Geometry check sheet. Reference: drawing and pictorial views, mm from the part's lowest x, y, z. Round coordinates to 2 decimals unless told otherwise and drop trailing zeros. Write each loop counter-clockwise with the first axis right and the second up, starting at its lowest first coordinate (ties: lowest second). Pieces come first, ordered by that corner, then holes. Notation, with made-up numbers: (-8, 82.5) -> (34, 82.5) arc R20 cw to (34, 103.5) -> close; hole circle Ø11 at (27.25, 69.25). An arc over 180 degrees is marked (long way). Answer as a JSON object with one key per item and string values. Group by question number.
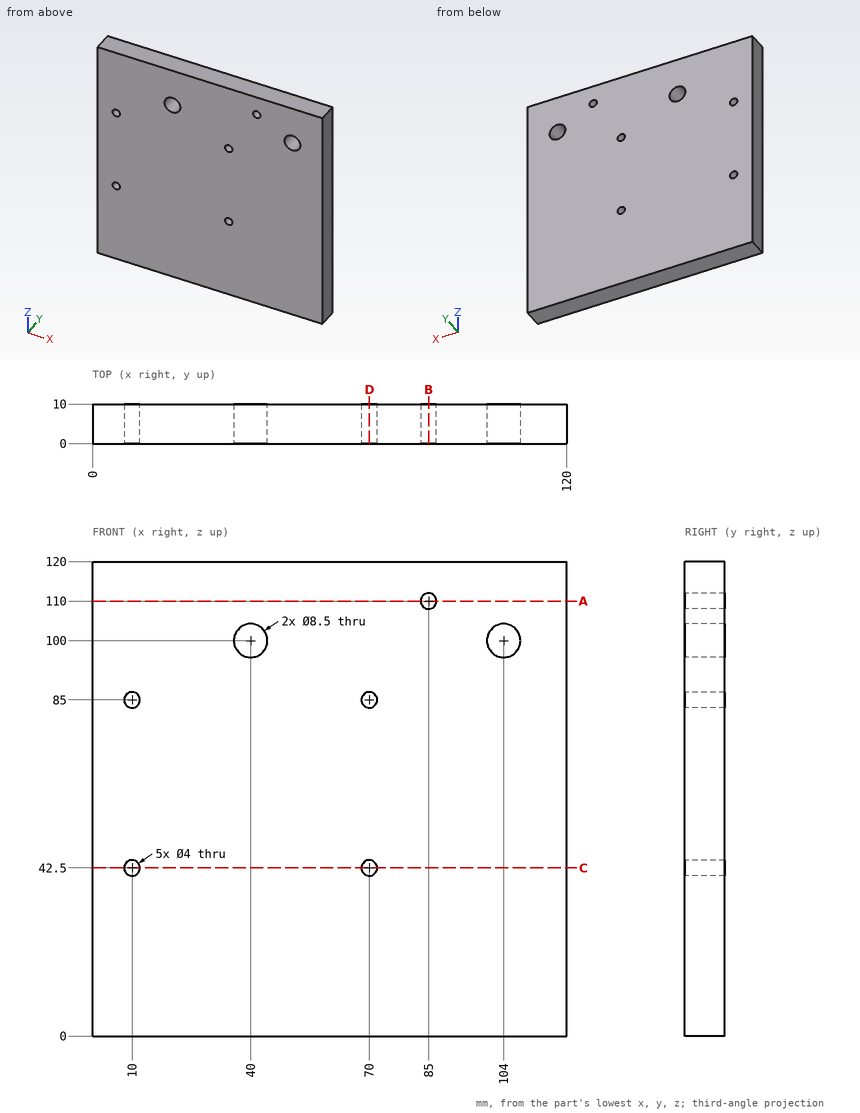
(1) Scan lines: line 1 along X through (y, z) = (6.5, 98); line 2 along Z through (x, y) = (105, 3.5); line 3 along Z through (x, y) = (107, 5). Record each from-to range of solid material in increasing order.
(2) Section check B-B on x = 85. Record the cut outline in (y, z), then the cut area to 3 significant figures.
(3) Section check C-C on z = 42.5. Record the cut outline in (x, y).
(4) Section check D-D on x = 70. Record the cut outline in (y, z).
(5) Go/stop test with a flat-tipped pin: pin 1 Ø3 at (x, z) = (10, 42.5) entering from +Y. Record where the tip stops, or that it passes through.
(6) Section check A-A on z = 110. Record the cut outline in (x, y).
Data:
{
 "1": {"line 1": "x = 0 to 36.25, 43.75 to 100.25, 107.75 to 120", "line 2": "z = 0 to 95.87, 104.13 to 120", "line 3": "z = 0 to 96.99, 103.01 to 120"},
 "2": {"outline": "(0, 0) -> (10, 0) -> (10, 108) -> (0, 108) -> close; (0, 112) -> (10, 112) -> (10, 120) -> (0, 120) -> close", "area": "1,160 mm²"},
 "3": {"outline": "(0, 0) -> (8, 0) -> (8, 10) -> (0, 10) -> close; (12, 0) -> (68, 0) -> (68, 10) -> (12, 10) -> close; (72, 0) -> (120, 0) -> (120, 10) -> (72, 10) -> close"},
 "4": {"outline": "(0, 0) -> (10, 0) -> (10, 40.5) -> (0, 40.5) -> close; (0, 44.5) -> (10, 44.5) -> (10, 83) -> (0, 83) -> close; (0, 87) -> (10, 87) -> (10, 120) -> (0, 120) -> close"},
 "5": {"pin 1": "passes through"},
 "6": {"outline": "(0, 0) -> (83, 0) -> (83, 10) -> (0, 10) -> close; (87, 0) -> (120, 0) -> (120, 10) -> (87, 10) -> close"}
}
